```python
from build123d import *


with BuildPart() as part:
    # Sketch1 → Revolve1 (revolve)
    with BuildSketch(Plane(origin=(0, 0, 0), x_dir=(0, 0, -1), z_dir=(1, 0, 0)), mode=Mode.PRIVATE) as revolve1_sk:
        with BuildLine():
            Line((0, 30.725), (0.5, 30.225))
            Line((0.5, 30.225), (8.6, 30.225))
            Line((8.6, 30.225), (9.1, 30.725))
            Line((9.1, 30.725), (9.1, 33.5))
            Line((9.1, 33.5), (8.6, 34))
            Line((8.6, 34), (5.4, 34))
            ThreePointArc((5.4, 34), (5.117157288, 34.117157288), (5, 34.4))
            Line((5, 34.4), (5, 38.06))
            Line((5, 38.06), (4, 39.06))
            Line((4, 39.06), (0.4, 39.06))
            ThreePointArc((0.4, 39.06), (0.117157288, 38.942842712), (0, 38.66))
            Line((0, 38.66), (0, 30.725))
        make_face()
    revolve(revolve1_sk.sketch.rotate(Axis((0, 0, 0), (0, 0, -1)), 90), axis=Axis((0, 0, 0), (0, 0, -1)))


solid = part.part
```
CAD build for the part. Positions are in the model's coordinates, mm. A direction names the side the tool comes from. Give positions to 0.01 mm unless a question says otherwise; leave off trailing zeros. Loops run counter-clockwise (first coordinate to the right, second up) from the corner with the lowest first, then second, coordinate; pieces in that order, holes last. Notation, with made-up numbers: (30.25, -23) - (35.25, -23) arc R27 ccw to (35.25, 2) - close; hole circle Ø10 at (70.5, 63). An arc over 180 degrees is marked (long way). Put each result on its own line as item: value.
Q1. Tool access for faces 4 (the face through (9, 34, -5)), 5 (the face through (-15, 27, -9.1)): list every direction of +Z, -Z, +X, -X, +Y, -Y with a clear straight run to the whole face (end or side of a thin tool).
Filled in:
face 4: -Z
face 5: -Z, +X, -X, +Y, -Y
Q2. Probe line 1 along Y through (x, z) = (0, -2.5) (3 decimals); line 2 along Y through (x, z) = (0, -5.5) (3 decimals); line 3 along X through (y, z) = (-25.5, -0.75). List the from-to ranges inside material, lowest first.
Filled in:
line 1: y = -39.06 to -30.225, 30.225 to 39.06
line 2: y = -34 to -30.225, 30.225 to 34
line 3: x = -29.59 to -16.23, 16.23 to 29.59
Q3. Slice it at A-A (x = 0). Give the cut face in (y, z) (3 decimals).
Filled in:
outline: (-39.06, -4) - (-38.06, -5) - (-34.4, -5) arc R0.4 cw to (-34, -5.4) - (-34, -8.6) - (-33.5, -9.1) - (-30.725, -9.1) - (-30.225, -8.6) - (-30.225, -0.5) - (-30.725, 0) - (-38.66, 0) arc R0.4 ccw to (-39.06, -0.4) - close; (30.225, -8.6) - (30.725, -9.1) - (33.5, -9.1) - (34, -8.6) - (34, -5.4) arc R0.4 cw to (34.4, -5) - (38.06, -5) - (39.06, -4) - (39.06, -0.4) arc R0.4 ccw to (38.66, 0) - (30.725, 0) - (30.225, -0.5) - close
Q4. Flat gauge pins, fed straight in: pin 1 (1.5 mm diameter, centred on y = -8.5, z = -7.5, fed in from +X); pin 2 (1.5 mm diameter, centred on x = 18.5, z = -8, fed in from +Y); pin 3 (23 mm diameter, centred on x = 8, y = -3, fed in from -Z); pin 4 (1 mm diameter, centred on y = -25, z = -6, fed in from -X). Where does each tip first touch, or does it go through?
Filled in:
pin 1: stops at x = 33.1
pin 2: stops at y = 29
pin 3: passes through
pin 4: stops at x = -23.57
Q5. Mould opens along Y. For faces 1 (the face through (-28.79, -26.4, -2.17)), 2 (the face through (28.83, -9.08, -4.61)), 3 (the face through (11, -29, 0)) say: pulls with the +Y half, pulls with the -Y half, needs draft (parallel to the pull), parting line crosses it, or undercut.
Filled in:
face 1: parting line crosses it
face 2: undercut
face 3: needs draft
